Verification items for this drawing (mm, ordinates from the low corner). Round coordinates to 2 decimals unless told otherwise and drop trailing zeros. Order: outer loops, then holes, each group sorted by start corner. A loop starts at its lowest first (then second) coordinate and runs counter-clockwise, first axis right, second up. Notation, with made-up numbers: (19, 3.5) -> (41, 3.5) arc R21 ccw to (41, 7.5) -> close; hole circle Ø2 at (-23.75, 49.25). An arc over 180 degrees is marked (long way). Return JSON: item names as keys, results as strings. Group by question number.
Item 1: Sectioned sample at D-D on y = 81. Record the cut outline in (x, z).
Item 2: Sectioned sample at C-C on y = 59.5. Record the cut outline in (x, z).
Item 3: Depth check by flat-ended pin: pin 1 Ø8 at (x, y) = (18, 78.5) entering from +Z (1 decimal); pin 2 Ø4 at (y, z) = (56.5, 28.5) entering from +X; pin 3 Ø3 at (x, z) = (44, 45) entering from +Y; pin 4 Ø4 at (x, y) = (38, 28.5) entering from +Z (1 decimal). Enter the tip coordinate at first touch or a pass-through.
Item 4: Sectioned sample at B-B on x = 29.5. Record the cut outline in (y, z), plus the area to 3 significant figures.
Item 5: Scan lines: probe 1 along Y at (x, z) = (32, 24); probe 2 along X at (y, z) = (55, 44.5); probe 3 along Z at (x, y) = (54, 48). Record each from-to range of solid material in increasing order. Write a range as from..to.
Item 6: Sectioned sample at A-A on z = 29.5. Record the cut outline in (x, y), plus the area to 3 significant figures.
Item 7: Draft check along Y on the marked faces 1, 2 and 3. Enter one of: pulls with the +Y half, pulls with the -Y half, needs draft (parallel to the pull), parting line crosses it, or undercut.
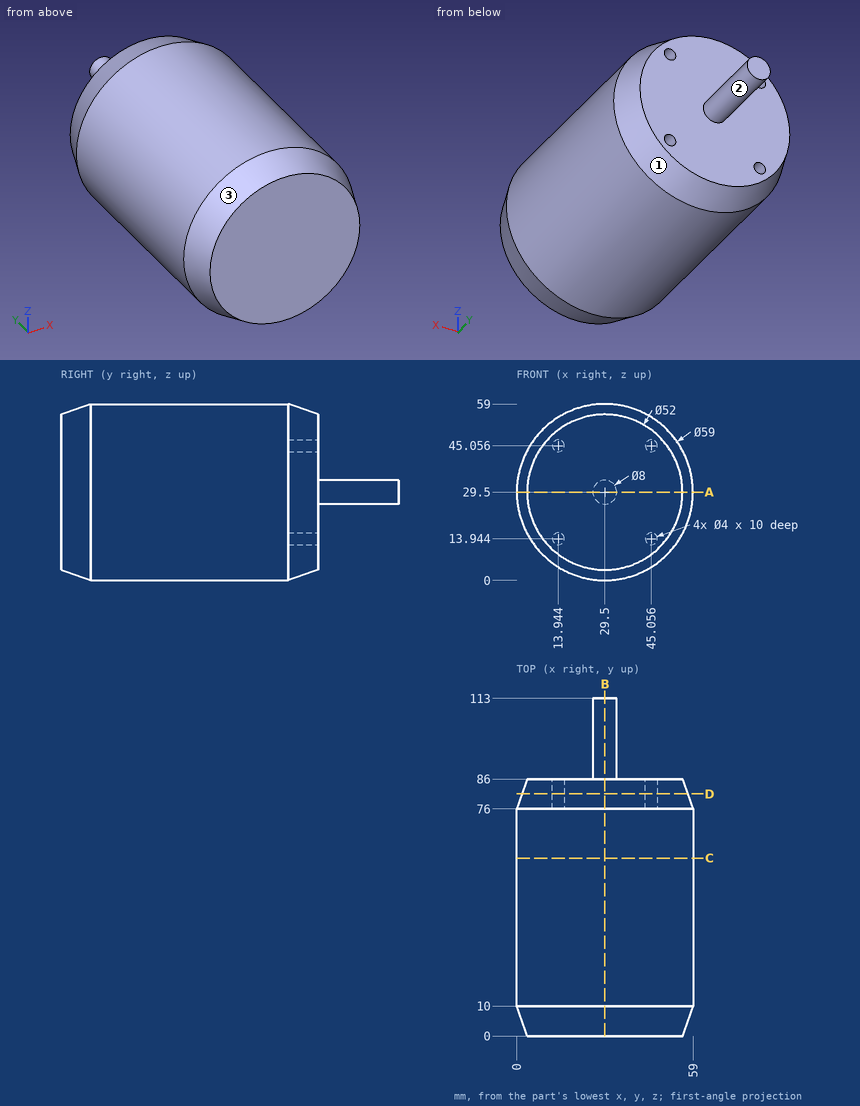
Recorded:
{
 "1": {"outline": "circle Ø55.5 at (29.5, 29.5); hole circle Ø4 at (13.94, 13.94); hole circle Ø4 at (13.94, 45.06); hole circle Ø4 at (45.06, 13.94); hole circle Ø4 at (45.06, 45.06)"},
 "2": {"outline": "circle Ø59 at (29.5, 29.5)"},
 "3": {"pin 1": "z = 57.8", "pin 2": "x = 59", "pin 3": "y = 86", "pin 4": "z = 58.3"},
 "4": {"outline": "(0, 3.5) -> (10, 0) -> (76, 0) -> (86, 3.5) -> (86, 25.5) -> (113, 25.5) -> (113, 33.5) -> (86, 33.5) -> (86, 55.5) -> (76, 59) -> (10, 59) -> (0, 55.5) -> close", "area": "5,220 mm²"},
 "5": {"probe 1": "0..86", "probe 2": "4.1..54.9", "probe 3": "13.07..45.93"},
 "6": {"outline": "(0, 10) -> (3.5, 0) -> (55.5, 0) -> (59, 10) -> (59, 76) -> (55.5, 86) -> (33.5, 86) -> (33.5, 113) -> (25.5, 113) -> (25.5, 86) -> (3.5, 86) -> (0, 76) -> close", "area": "5,220 mm²"},
 "7": {"face 1": "pulls with the +Y half", "face 2": "needs draft", "face 3": "pulls with the -Y half"}
}
